The listing builds one solid part. Answer for the finished solid, in the listing's coordinates (mm). Face numbers are marked on the shaded views. Coordinates: 2 decimals unless noted, no trailing zeros. Loops run counter-clockwise (first coordinate to the right, second up) from the corner with the lowest first, then second, coordinate; pieces in that order, holes last. Notation, with made-up numbers: M 10,19.25 L 16,19.25 A7 cw 16,23.25 Z; hole C 89.25,-8.75 d9. An arc over 180 degrees is marked long. Return JSON: item names as keys, results as strings. Group by question number.
1. Given P1, Ø11.5, axis at x = 0, y = 0, coming from the -Z side; P2, Ø3, axis at x = 0.5, z = 5.5, coming from the +Y side; P3, Ø2, axis at y = 22, z = 2.5, coming from the +X side, each flat-ended and moving along its own axis, determine where each tip first touches the part or whether it passes through.
2. The mould has two halves that part along Y. Classify the marked faces 1, 2 and 3: pulls with the +Y half, pulls with the -Y half, needs draft (parallel to the pull), parting line crosses it, or undercut.
3. Section C-C (z = 5.5) is taken. Count the separate pieces of the cut face and the enclosed holes in it, then the cut area to 3 significant figures.
4. Section D-D (y = 0) is taken. Write down the section's boundary in (x, z), then the cut area to 3 significant figures.
5. Section B-B (y = 63.5) is taken. Write down the section's boundary in (x, z) (1 decimal).
6. Straight lines are drawn through the part: L1, parallel to Y at x = 0, z = 1.75 (3 decimals); L2, parallel to X at y = 62, z = 3.5; L3, parallel to Y at x = -50, z = 7.25. For each, find the intervals that lie inside material, in ascending order. Write a range as from..to.
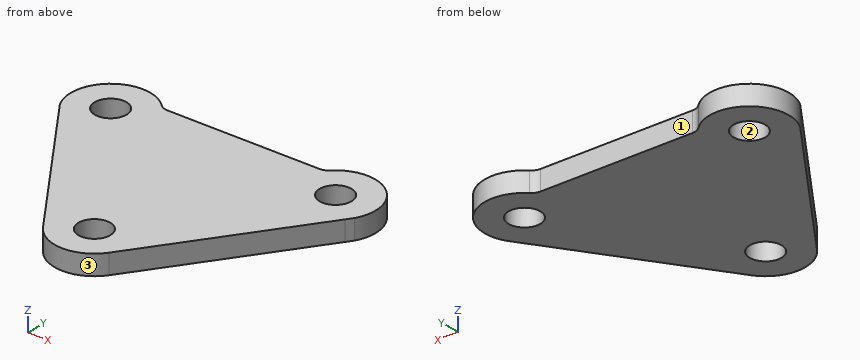
```python
from build123d import *

# Parameters (mm, degrees)
F0_R     = 6.35
F1_DEPTH = 7.9375


with BuildPart() as f1:
    # F0 (on Top) → F1 (new body)
    with BuildSketch(Plane.XY):
        with BuildLine():
            Line((-56.530945, 53.201145), (-13.013914, -9.091406))
            ThreePointArc((-13.013914, -9.091406), (0, -15.875), (13.013914, -9.091406))
            Line((13.013914, -9.091406), (56.530945, 53.201145))
            Line((56.530945, 53.201145), (58.276649, 55.700037))
            ThreePointArc((58.276649, 55.700037), (54.115532, 76.093376), (33.339815, 74.839286))
            ThreePointArc((33.339815, 74.839286), (31.806815, 73.831853), (30.006759, 73.478571))
            Line((30.006759, 73.478571), (-30.006759, 73.478571))
            ThreePointArc((-30.006759, 73.478571), (-31.806815, 73.831853), (-33.339815, 74.839286))
            ThreePointArc((-33.339815, 74.839286), (-54.115532, 76.093376), (-58.276649, 55.700037))
            Line((-58.276649, 55.700037), (-56.530945, 53.201145))
        make_face()
        Circle(F0_R, mode=Mode.SUBTRACT)
        with Locations((-44.45, 63.5)):
            Circle(F0_R, mode=Mode.SUBTRACT)
        with Locations((44.45, 63.5)):
            Circle(F0_R, mode=Mode.SUBTRACT)
    extrude(amount=F1_DEPTH)


solid = f1.part
```
Worked out:
{
 "1": {"P1": "through", "P2": "y = 73.48", "P3": "x = 35.43"},
 "2": {"face 1": "pulls with the +Y half", "face 2": "undercut", "face 3": "pulls with the -Y half"},
 "3": {"separate pieces": "1", "enclosed holes": "3", "area": "6,680 mm^2"},
 "4": {"outline": "M -19.37,0 L -6.35,0 L -6.35,7.94 L -19.37,7.94 Z; M 6.35,0 L 19.37,0 L 19.37,7.94 L 6.35,7.94 Z", "area": "207 mm^2"},
 "5": {"outline": "M -60.3,0 L -50.8,0 L -50.8,7.9 L -60.3,7.9 Z; M -38.1,0 L 38.1,0 L 38.1,7.9 L -38.1,7.9 Z; M 50.8,0 L 60.3,0 L 60.3,7.9 L 50.8,7.9 Z"},
 "6": {"L1": "-15.875..-6.35, 6.35..73.479", "L2": "-60.25..-50.62, -38.28..38.28, 50.62..60.25", "L3": "43.85..60.41, 66.59..78.37"}
}
